from build123d import *

# Parameters (mm, degrees)
SKETCH1_W               = 96.52
SKETCH1_H               = 44.45
BOSS_EXTRUDE1_DEPTH     = 6.096
CUT_EXTRUDE1_REACH      = 108.961
SKETCH2_R               = 11.50874
CUT_EXTRUDE2_REACH      = 108.438
SKETCH3_R               = 3.3782
CUT_EXTRUDE3_REACH      = 108.961
SKETCH7_W               = 12.7635
SKETCH7_H               = 12.192
CUT_EXTRUDE5_DEPTH      = 104.946532487
FILLET1_R               = 11.43
CUT_EXTRUDE9_REACH      = 97.016
CUT_EXTRUDE9_END_RADIUS = 11.50874
SKETCH11_R              = 2.0193
SKETCH12_R              = 6.35
CUT_EXTRUDE10_DEPTH     = 96.601248341


with BuildPart() as part:
    # Sketch1 → Boss-Extrude1 (new, symmetric)
    with BuildSketch(Plane.XY):
        with Locations((48.26, -22.225)):
            Rectangle(SKETCH1_W, SKETCH1_H)
    extrude(amount=BOSS_EXTRUDE1_DEPTH, both=True)

    # Sketch2 → Cut-Extrude1 (cut, up to next)
    with BuildSketch(Plane.XY.offset(6.096), mode=Mode.PRIVATE) as cut_extrude1_sk1:
        with Locations((22.225, -22.225)):
            Circle(SKETCH2_R)
    cut_extrude1_tool1 = extrude(cut_extrude1_sk1.sketch, amount=-CUT_EXTRUDE1_REACH, mode=Mode.PRIVATE) & part.part
    add(cut_extrude1_tool1.solids().sort_by_distance((22.225, -22.225, 6.096))[0], mode=Mode.SUBTRACT)

    # Sketch3 → Cut-Extrude2 (cut, up to next)
    with BuildSketch(Plane(origin=(0, 0, 0), x_dir=(1, 0, 0), z_dir=(0, 1, 0)), mode=Mode.PRIVATE) as cut_extrude2_sk1:
        with Locations(Location((77.4065, -0.254, 0), (0, 0, 270))):
            Circle(SKETCH3_R)
    cut_extrude2_tool1 = extrude(cut_extrude2_sk1.sketch, amount=-CUT_EXTRUDE2_REACH, mode=Mode.PRIVATE) & part.part
    add(cut_extrude2_tool1.solids().sort_by_distance((77.4065, 0, 0.254))[0], mode=Mode.SUBTRACT)

    # Sketch4 → Cut-Extrude3 (cut, up to next)
    with BuildSketch(Plane.XY.offset(6.096), mode=Mode.PRIVATE) as cut_extrude3_sk1:
        with BuildLine():
            Line((48.895, 6.35), (96.52, 6.35))
            ThreePointArc((96.52, 6.35), (102.87, 0), (96.52, -6.35))
            Line((96.52, -6.35), (48.895, -6.35))
            ThreePointArc((48.895, -6.35), (42.545, 0), (48.895, 6.35))
        make_face()
    cut_extrude3_tool1 = extrude(cut_extrude3_sk1.sketch, amount=-CUT_EXTRUDE3_REACH, mode=Mode.PRIVATE) & part.part
    # Sketch4 → Cut-Extrude3 (cut, up to next)
    with BuildSketch(Plane.XY.offset(6.096), mode=Mode.PRIVATE) as cut_extrude3_sk2:
        with BuildLine():
            Line((45.72, -34.925), (45.72, -44.45))
            Line((45.72, -44.45), (55.245, -44.45))
            Line((55.245, -44.45), (96.52, -44.45))
            ThreePointArc((96.52, -44.45), (106.045, -34.925), (96.52, -25.4))
            Line((96.52, -25.4), (55.245, -25.4))
            ThreePointArc((55.245, -25.4), (48.509807909, -28.189807909), (45.72, -34.925))
        make_face()
    cut_extrude3_tool2 = extrude(cut_extrude3_sk2.sketch, amount=-CUT_EXTRUDE3_REACH, mode=Mode.PRIVATE) & part.part
    add(cut_extrude3_tool1.solids().sort_by_distance((72.7075, 0, 6.096))[0], mode=Mode.SUBTRACT)
    add(cut_extrude3_tool2.solids().sort_by_distance((75.382091, -35.05704, 6.096))[0], mode=Mode.SUBTRACT)

    # Sketch7 → Cut-Extrude5 (cut, through all)
    with BuildSketch(Plane(origin=(0, -6.35, 0), x_dir=(1, 0, 0), z_dir=(0, 1, 0))):
        with Locations((90.13825, 0)):
            Rectangle(SKETCH7_W, SKETCH7_H)
    extrude(amount=-CUT_EXTRUDE5_DEPTH, mode=Mode.SUBTRACT)

    # Fillet1
    fillet1_edges = [part.edges().sort_by_distance(p)[0] for p in [
        (42.545, 0, 0),
        (45.72, -44.45, 0),
        (0, -44.45, 0),
        (0, 0, 0),
    ]]
    fillet(fillet1_edges, radius=FILLET1_R)

    # Cut-Extrude9: up to this cylinder (the profile starts outside it)
    cut_extrude9_end = Plane(origin=(22.225, -22.225, 0), z_dir=(0, 0, 1)) * Cylinder(CUT_EXTRUDE9_END_RADIUS, 218.04948, mode=Mode.PRIVATE)
    # Sketch11 → Cut-Extrude9 (cut, up to the surface)
    with BuildSketch(Plane.ZY, mode=Mode.PRIVATE) as cut_extrude9_sk1:
        with Locations(Location((0, -22.225, 0), (0, 0, 270))):
            Circle(SKETCH11_R)
    cut_extrude9_tool1 = extrude(cut_extrude9_sk1.sketch, amount=-CUT_EXTRUDE9_REACH, mode=Mode.PRIVATE) - cut_extrude9_end
    add(cut_extrude9_tool1.solids().sort_by_distance((0, -22.225, 0))[0], mode=Mode.SUBTRACT)

    # Sketch12 → Cut-Extrude10 (cut, through all)
    with BuildSketch(Plane.XY.offset(6.096)):
        with Locations((44.45, -16.66875)):
            Circle(SKETCH12_R)
        with BuildLine():
            Line((17.78, -3.175), (11.43, -3.175))
            ThreePointArc((11.43, -3.175), (5.592833521, -5.592833521), (3.175, -11.43))
            Line((3.175, -11.43), (3.175, -17.78))
            ThreePointArc((3.175, -17.78), (3.546974388, -18.678025612), (4.445, -19.05))
            Line((4.445, -19.05), (6.902996378, -19.05))
            ThreePointArc((6.902996378, -19.05), (7.665727307, -18.795451392), (8.122706904, -18.133844929))
            ThreePointArc((8.122706904, -18.133844929), (11.842027873, -11.842027873), (18.133844929, -8.122706904))
            ThreePointArc((18.133844929, -8.122706904), (18.795451392, -7.665727307), (19.05, -6.902996378))
            Line((19.05, -6.902996378), (19.05, -4.445))
            ThreePointArc((19.05, -4.445), (18.678025612, -3.546974388), (17.78, -3.175))
        make_face()
        with BuildLine():
            Line((26.67, -41.275), (33.718820715, -41.275))
            ThreePointArc((33.718820715, -41.275), (34.892147722, -40.491007959), (34.616846327, -39.106974388))
            Line((34.616846327, -39.106974388), (30.814228632, -35.304356693))
            ThreePointArc((30.814228632, -35.304356693), (30.094903373, -34.945017527), (29.303943585, -35.089710572))
            ThreePointArc((29.303943585, -35.089710572), (27.844224023, -35.791006847), (26.316155071, -36.327293096))
            ThreePointArc((26.316155071, -36.327293096), (25.654548608, -36.784272693), (25.4, -37.547003622))
            Line((25.4, -37.547003622), (25.4, -40.005))
            ThreePointArc((25.4, -40.005), (25.771974388, -40.903025612), (26.67, -41.275))
        make_face()
        with BuildLine():
            Line((34.616846327, -5.343025612), (30.814228632, -9.145643307))
            ThreePointArc((30.814228632, -9.145643307), (30.094903373, -9.504982473), (29.303943585, -9.360289428))
            ThreePointArc((29.303943585, -9.360289428), (27.844224023, -8.658993153), (26.316155071, -8.122706904))
            ThreePointArc((26.316155071, -8.122706904), (25.654548608, -7.665727307), (25.4, -6.902996378))
            Line((25.4, -6.902996378), (25.4, -4.445))
            ThreePointArc((25.4, -4.445), (25.771974388, -3.546974388), (26.67, -3.175))
            Line((26.67, -3.175), (33.718820715, -3.175))
            ThreePointArc((33.718820715, -3.175), (34.892147722, -3.958992041), (34.616846327, -5.343025612))
        make_face()
        with BuildLine():
            Line((11.43, -41.275), (17.78, -41.275))
            ThreePointArc((17.78, -41.275), (18.678025612, -40.903025612), (19.05, -40.005))
            Line((19.05, -40.005), (19.05, -37.547003622))
            ThreePointArc((19.05, -37.547003622), (18.795451392, -36.784272693), (18.133844929, -36.327293096))
            ThreePointArc((18.133844929, -36.327293096), (11.842027873, -32.607972127), (8.122706904, -26.316155071))
            ThreePointArc((8.122706904, -26.316155071), (7.665727307, -25.654548608), (6.902996378, -25.4))
            Line((6.902996378, -25.4), (4.445, -25.4))
            ThreePointArc((4.445, -25.4), (3.546974388, -25.771974388), (3.175, -26.67))
            Line((3.175, -26.67), (3.175, -33.02))
            ThreePointArc((3.175, -33.02), (5.592833521, -38.857166479), (11.43, -41.275))
        make_face()
    extrude(amount=-CUT_EXTRUDE10_DEPTH, mode=Mode.SUBTRACT)


solid = part.part
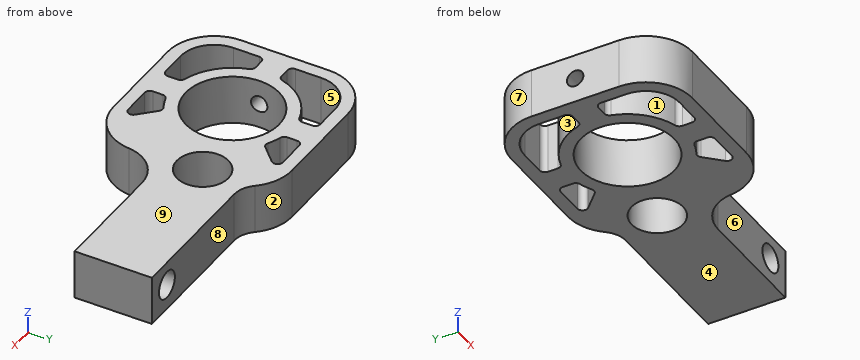
Geometry: final body of the model. Coordinates: model frame, mm. Face numbers are marked on the shaded views. A direction names the side the tool comes from. Coordinates: 2 decimals unless noted, no trailing zeros. Order: outer loops, then holes, each group sorted by start corner. A loop starts at its lowest first (then second) coordinate and runs counter-clockwise, first axis right, second up.
1) Section B-B (x = 48). Return loops of the section in (y, z), then the cut area to 3 significant figures.
Result sheet:
outline: (-28.74, -6.1) - (-21.93, -6.1) - (-21.93, 6.1) - (-28.74, 6.1) - close; (-11.4, -6.1) - (-6.29, -6.1) - (-6.29, 6.1) - (-11.4, 6.1) - close
area: 145 mm2
2) Section A-A (x = 12.5). Return loops of the section in (y, z) (3 decimals).
Result sheet:
outline: (-44.45, -6.096) - (-41.275, -6.096) - (-41.275, 6.096) - (-44.45, 6.096) - close; (-33.227, -6.096) - (-28.379, -6.096) - (-28.379, 6.096) - (-33.227, 6.096) - close; (-16.071, -6.096) - (-11.223, -6.096) - (-11.223, 6.096) - (-16.071, 6.096) - close; (-3.175, -6.096) - (0, -6.096) - (0, 6.096) - (-3.175, 6.096) - close
3) Set-up query: the marked faces 5, 6, 7, 8 and 9. Return all of +Z, -Z, +X, -X, +Y, -Y with unobstructed straight access to the full face (end or side cutting, diameter ignored); none if empty.
Result sheet:
face 5: +Z, -Z
face 6: +Z, -Z, +X, -Y
face 7: +Z, -Z, -X, +Y
face 8: +Z, -Z, +X, +Y
face 9: +Z, +X, -X, +Y, -Y
4) Section D-D (x = 75.5). Return loops of the section in (y, z).
Result sheet:
outline: (-25.4, -6.1) - (-6.35, -6.1) - (-6.35, -2.53) - (-25.4, -2.53) - close; (-25.4, 3.04) - (-6.35, 3.04) - (-6.35, 6.1) - (-25.4, 6.1) - close
5) Draft query along Y for the marked faces 1, 2, 3 and 4. Return one class per face: released by +Y, released by -Y, zero draft, split by the parting line, or undercut.
Result sheet:
face 1: undercut
face 2: released by +Y
face 3: undercut
face 4: zero draft
6) Ray query, probe 1 along X at (y, z) = (-24.5, 2); probe 2 along Y at (x, z) = (32, 2.75) (3 decimals); probe 3 along X at (y, z) = (-22.5, -4.75). Return the intervals inside material, ascending.
Result sheet:
probe 1: x = 0 to 10.94, 33.51 to 74.51, 80.3 to 83.76
probe 2: y = -44.45 to -41.275, -36.49 to -28.3, -16.15 to -7.96, -3.175 to 0
probe 3: x = 0 to 10.72, 33.73 to 41.94, 46.96 to 83.76
7) Section C-C (z = 0). Give the number of separate pieces and of enclosed holes in the cut face, then the cut area to 3 significant figures.
Result sheet:
separate pieces: 2
enclosed holes: 5
area: 1,570 mm2
8) First-contact query: P1, Ø2, axis at y = -6, z = -0.5, coming from the -X side; P2, Ø2, axis at y = -39, z = 0.5, coming from the +X side; P3, Ø6, axis at x = 57, z = -2, coming from the +Y side. Flat tips, straight axial feed; report the tip coordinate or a pass-through.
Result sheet:
P1: stops at x = 0.89
P2: stops at x = 44.66
P3: stops at y = -6.35
